The figure shows three views and two pictorial views of one solid part (mm, origin at its lowest corner). Answer the questions. A direction names the side the tool comes from. Give positions to 0.01 mm unless a question says otherwise; leave off trailing zeros. Loops run counter-clockwise (first coordinate to the right, second up) from the corner with the lowest first, then second, coordinate; pieces in that order, holes last.
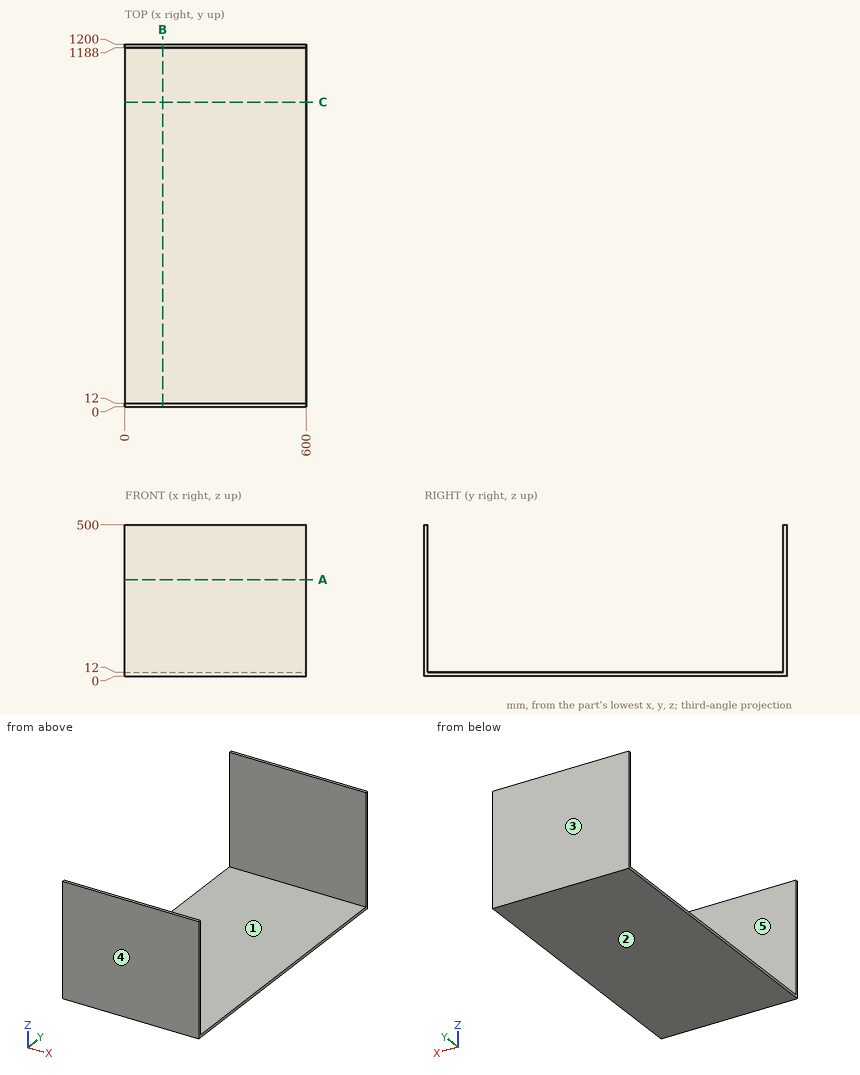
Q1. Section B-B on x = 124.5 is taken. Give the vertices of the cut face in (y, z), plus the area to 3 significant figures.
Q2. Given pin 1 (8 mm diameter, centred on x = 487, y = 270.5, fed in from +Z), flat-ended and moving along its own axis, determine where the tip first touches the part or whether it passes through.
Q3. Consider line 1 along Y through (x, z) = (281, 329.5); line 2 along Z through (x, y) = (513.5, 618). Determine where each line is inside the solid, lowest interval first.
Q4. Which of the six approach directions +Z, -Z, +X, -X, +Y, -Y give full straight-line access (tool end or side, diameter ignored) to the marked faces 1 and 2?
Q5. Section C-C on y = 1007.5 is taken. Give the vertices of the cut face in (x, z).
Q6. Determine the mould class of the marked faces 3, 4 and 5 for opening direction Y: +Y half, -Y half, draft (parallel to the pull), parting line (faces both ways), or undercut.
Q7. Section A-A on z = 319 is taken. Give the vertices of the cut face in (x, y), plus the area to 3 significant figures.
Check result:
1. outline: (0, 0) - (1200, 0) - (1200, 500) - (1188, 500) - (1188, 12) - (12, 12) - (12, 500) - (0, 500) - close
1. area: 26,100 mm2
2. pin 1: stops at z = 12
3. line 1: y = 0 to 12, 1188 to 1200
3. line 2: z = 0 to 12
4. face 1: +Z, +X, -X
4. face 2: -Z, +X, -X, +Y, -Y
5. outline: (0, 0) - (600, 0) - (600, 12) - (0, 12) - close
6. face 3: +Y half
6. face 4: -Y half
6. face 5: undercut
7. outline: (0, 0) - (600, 0) - (600, 12) - (0, 12) - close; (0, 1188) - (600, 1188) - (600, 1200) - (0, 1200) - close
7. area: 14,400 mm2
